Autodesk Inventor part; units mm, degrees
ref_plane "YZ Plane" through (0, 0, 0) normal (1, 0, 0) x (0, 1, 0)
ref_plane "XZ Plane" through (0, 0, 0) normal (0, 1, 0) x (-1, 0, 0)
ref_plane "XY Plane" through (0, 0, 0) normal (0, 0, 1) x (1, 0, 0)
sketch "Sketch1" plane through (0, 0, 0) normal (0, 0, 1) x (1, 0, 0)
  line L0 (-20.5, -40) -> (-20.5, -10.7426)
  line L1 (-9.7574, 0) -> (9.7574, 0)
  line L2 (20.5, -10.7426) -> (20.5, -40)
  line L3 (20.5, -40) -> (23.5, -40)
  line L4 (23.5, -40) -> (23.5, -9.5)
  line L5 (-20.5, -40) -> (-23.5, -40)
  line L6 (-23.5, -40) -> (-23.5, -9.5)
  line L7 (-11, 3) -> (11, 3)
  line L8 (-11, 3) -> (-23.5, -9.5)
  line L9 (-9.7574, 0) -> (-20.5, -10.7426)
  line L10 (11, 3) -> (23.5, -9.5)
  line L11 (9.7574, 0) -> (20.5, -10.7426)
  point P0 (0, 0)
extrude "Extrusion1" add sketch "Sketch1" along normal blind 22
sketch "Sketch2" plane through (23.5, -40, 0) normal (1, 0, 0) x (0, 0, -1)
  line L0 (-22, 30.5) -> (-22, 0)
  line L1 (0, 0) -> (-22, 0)
  line L2 (0, 0) -> (0, 30.5)
  line L3 (0, 30.5) -> (-22, 30.5)
  arc A0 (-22, 11) -> (0, 11) centre (-11, 11) ccw
  line L4 (-22, 29.2574) -> (-22, 0)
  line L5 (-22, 11) -> (-22, -1)
  line L6 (-22, -1) -> (0, -1)
  line L7 (0, -1) -> (0, 11)
  line L8 (0, 0) -> (0, 29.2574)
  circle A1 centre (-11, 11) radius 4.5
  line L9 (-15.5, 11) -> (-15.5, -1)
  line L10 (-6.5, 11) -> (-6.5, -1)
  point P0 (0, 40)
  dimension "d2" = 22
  dimension "d3" = 11
  dimension "d4" = 9
extrude "Extrusion2" cut sketch "Sketch2" against normal through all contours A0 L9 L1 L0 | L1 L9 L6 L5 | L9 A1 L10 A0 | A0 L1 L9 | L2 L1 L10 A0 | L1 L10 L6 L9 | A0 L10 L1 | A1 | L7 L6 L10 L1
sketch "Sketch3" plane through (-9.7574, 0, 0) normal (0, -1, 0) x (1, 0, 0)
  circle A0 centre (9.7574, 11) radius 5
  point P0 (9.7574, 0)
  dimension "d7" = 10
extrude "Extrusion3" cut sketch "Sketch3" against normal through all
sketch "Sketch4" plane through (23.5, -9.5, 22) normal (1, 0, 0) x (0, 0, -1)
  arc A0 (15.5, -29.5374) -> (22, -19.5) centre (11, -19.5) ccw
  line L0 (11, -19.5) -> (18.853, -16.2472)
  line L1 (11, -19.5) -> (19.5, -19.5) construction
  circle A1 centre (18.853, -16.2472) radius 1
  point P0 (22, 9.5)
  dimension "d10" = 8.5
  dimension "d11" = 22.5
  dimension "d12" = 2
extrude "Extrusion4" cut sketch "Sketch4" against normal through all
pattern_circular "Circular Pattern1" count 8 over 360 about axis through (23.5, -29, 11) along (-1, 0, 0) of "Extrusion4"
sketch "Sketch5" plane through (-9.7574, 0, 0) normal (0, -1, 0) x (1, 0, 0)
  circle A0 centre (9.7574, 11) radius 5
  circle A1 centre (9.7574, 19.5) radius 1
  point P0 (9.7574, 0)
  dimension "d18" = 2
  dimension "d19" = 8.5
extrude "Extrusion5" cut sketch "Sketch5" against normal through all contours A1
pattern_circular "Circular Pattern2" count 8 over 360 about axis through (0, 0, 11) along (0, 1, 0) of "Extrusion5"
properties part number "Waistline" material "Aluminum-6061"
Can you work these out from the model? Positions are in its coordinate system, mm. A direction names the side the tool comes from. Give positions to 0.01 mm unless a question says otherwise; leave off trailing zeros. Loops run counter-clockwise (first coordinate to the right, second up) from the corner with the lowest first, then second, coordinate; pieces in that order, holes last. Notation, with made-up numbers: (-23, 63.25) - (27, 63.25) arc R9 cw to (27, 79.25) - close; hole circle Ø8 at (34.5, 10). An arc over 180 degrees is marked (long way). Return JSON: item names as keys, results as strings.
1. I want a section at B-B on y = -35.5. Please give me the cut outline in (x, z), and give its area (3 significant figures).
Output values:
{"outline": "(-23.5, 2.13) - (-20.5, 2.13) - (-20.5, 6.5) - (-23.5, 6.5) - close; (-23.5, 15.5) - (-20.5, 15.5) - (-20.5, 19.87) - (-23.5, 19.87) - close; (20.5, 2.13) - (23.5, 2.13) - (23.5, 6.5) - (20.5, 6.5) - close; (20.5, 15.5) - (23.5, 15.5) - (23.5, 19.87) - (20.5, 19.87) - close", "area": "52.5 mm²"}
2. I want a section at A-A on z = 11. Please give me the cut outline in (x, y).
Output values:
{"outline": "(-23.5, -24.5) - (-20.5, -24.5) - (-20.5, -10.74) - (-9.76, 0) - (-9.5, 0) - (-9.5, 3) - (-11, 3) - (-23.5, -9.5) - close; (-7.5, 0) - (-5, 0) - (-5, 3) - (-7.5, 3) - close; (5, 0) - (7.5, 0) - (7.5, 3) - (5, 3) - close; (9.5, 0) - (9.76, 0) - (20.5, -10.74) - (20.5, -24.5) - (23.5, -24.5) - (23.5, -9.5) - (11, 3) - (9.5, 3) - close"}
3. If I drill on line 1 (Z direction, x = 0, y = 1.75); line 2 (X direction, y = -13, z = 19.75); line 3 (Y direction, x = -2.5, z = 18.25), over which ranges is the centre line in solid material (lowest first)?
Output values:
{"line 1": "z = 0 to 1.5, 3.5 to 6, 16 to 18.5, 20.5 to 22", "line 2": "x = -23.5 to -20.5, 20.5 to 23.5", "line 3": "y = 0 to 3"}
4. I'm going to push flat-ended pins straight in: pin 1 Ø1.5 at (x, y) = (22, -33) entering from -Z; pin 2 Ø10 at (y, z) = (-4, 9) entering from +X; pin 3 Ø0.9 at (x, y) = (-22.5, -36) entering from -Z. Where does each tip first touch, or does it pass through?
Output values:
{"pin 1": "stops at z = 0.49", "pin 2": "stops at x = 23", "pin 3": "stops at z = 2.16"}
5. For faces 1 (the face through (-20.5, -22, 11)), 2 (the face through (-21.98, -25.21, 18.01)), 3 (the face through (-22, -34, 15.5)), which set-ups out of +Z, -Z, +X, -X, +Y, -Y let a thin tool reach every point of the face, with its end or its side?
Output values:
{"face 1": "+Z, -Z, -Y", "face 2": "+X, -X", "face 3": "+X, -X, -Y"}
6. I want a section at D-D on x = -6. Please give me the cut outline in (y, z), and give its area (3 significant figures).
Output values:
{"outline": "(0, 0) - (3, 0) - (3, 3.99) - (0, 3.99) - close; (0, 5.99) - (3, 5.99) - (3, 16.01) - (0, 16.01) - close; (0, 18.01) - (3, 18.01) - (3, 22) - (0, 22) - close", "area": "54.0 mm²"}
7. We'd pull the mould along X, two halves only. Please class faces 4 (the face through (22, -34, 6.5)), 5 (the face through (20.5, -22, 11)), 6 (the face through (-17, -3, 11)): +X half, -X half, draft (parallel to the pull), parting line (faces both ways), or undercut.
Output values:
{"face 4": "draft", "face 5": "undercut", "face 6": "-X half"}
8. I want a section at C-C on x = 0. Please give me the cut outline in (y, z), and give its area (3 significant figures).
Output values:
{"outline": "(0, 0) - (3, 0) - (3, 1.5) - (0, 1.5) - close; (0, 3.5) - (3, 3.5) - (3, 6) - (0, 6) - close; (0, 16) - (3, 16) - (3, 18.5) - (0, 18.5) - close; (0, 20.5) - (3, 20.5) - (3, 22) - (0, 22) - close", "area": "24.0 mm²"}
